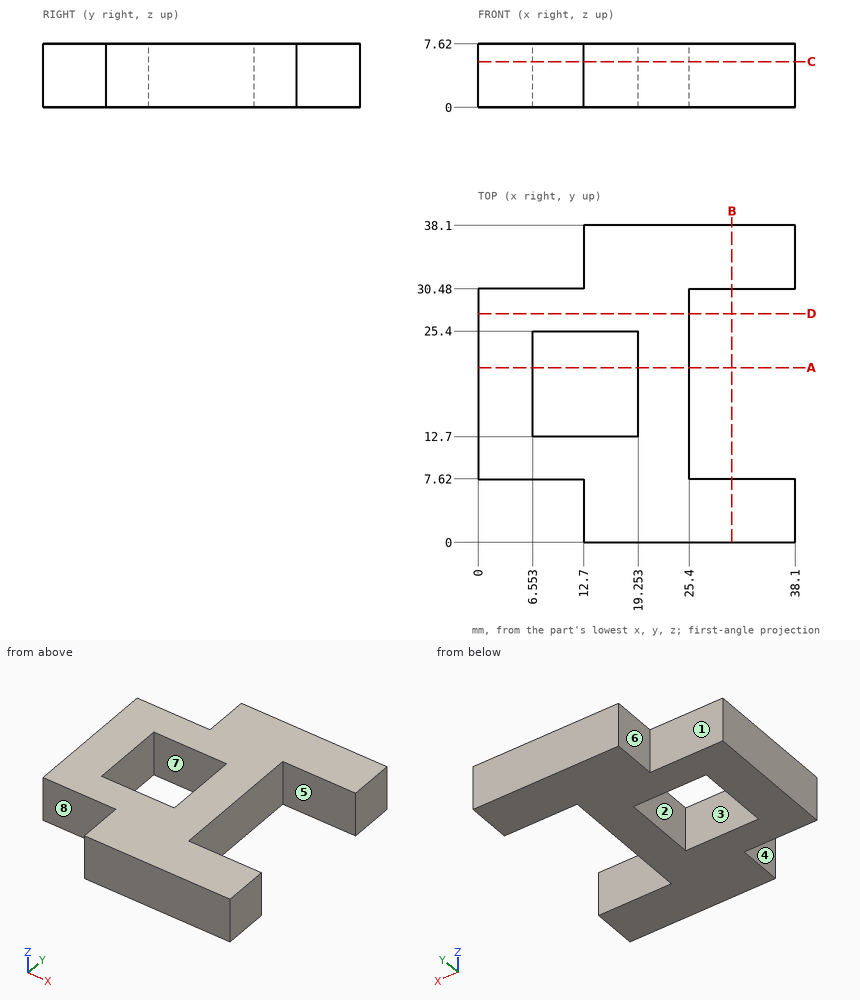
Input: dimensioned drawing with shaded views. Units: mm. Origin: part minimum x, y, z. A direction names the side the tool comes from. Give positions to 0.01 mm unless a question says otherwise; leave off trailing zeros. Loops run counter-clockwise (first coordinate to the right, second up) from the corner with the lowest first, then second, coordinate; pieces in that order, holes last. Notation, with made-up numbers: M 18,-10 L 63,-10 A33 ccw 63,23 Z; hole C 82,42.5 d11. An arc over 180 degrees is marked long. Put each result on its own line as item: value. Start each with the question number.
1) Ray query, line 1 along Y through (x, z) = (9, 6); line 2 along X through (y, z) = (13.5, 5); line 3 along Y through (x, z) = (36, 4). Return the intervals inside material, ascending.
2) Contact query for flat-ended pins moving along their axis: pin 1 (10 mm diameter, centred on x = 24, y = 8.5, fed in from -Z); pin 2 (2.5 mm diameter, centred on x = 6, z = 4.5, fed in from -Y); pin 3 (2.5 mm diameter, centred on y = 21.5, z = 2.5, fed in from +X); pin 4 (4 mm diameter, centred on y = 5.5, z = 5.5, fed in from -X). Output: stop coordinate, or through.
3) Access query for the marked faces 5, 6, 7 and 8. Directions: +Z, -Z, +X, -X, +Y, -Y. A direction counts if a zero-diameter tool reaches every point of the face in a straight line with its end or side. Return the directions, or none.
4) Pull-direction query (X, two-part tool) for the marked faces 1, 2, 3 and 4; classes: pulls with the +X half, pulls with the -X half, needs draft (parallel to the pull), parting line crosses it, or undercut.
5) Cut plane B-B (x = 30.5). Output: boundary loops of the cut face in (y, z), then the cut area to 3 significant figures.
6) Cut plane D-D (y = 27.5). Output: boundary loops of the cut face in (x, z).
7) Cut plane A-A (y = 21). Output: boundary loops of the cut face in (x, z), then the cut area to 3 significant figures.
8) Cut plane C-C (z = 5.5). Output: boundary loops of the cut face in (x, y).
Verdict:
1. line 1: 7.62 to 12.7, 25.4 to 30.48
1. line 2: 0 to 6.55, 19.25 to 25.4
1. line 3: 0 to 7.62, 30.48 to 38.1
2. pin 1: z = 0
2. pin 2: y = 7.62
2. pin 3: x = 25.4
2. pin 4: x = 12.7
3. face 5: +Z, -Z, +X
3. face 6: +Z, -Z, -X, +Y
3. face 7: +Z, -Z
3. face 8: +Z, -Z, -X, -Y
4. face 1: needs draft
4. face 2: undercut
4. face 3: undercut
4. face 4: pulls with the -X half
5. outline: M 0,0 L 7.62,0 L 7.62,7.62 L 0,7.62 Z; M 30.48,0 L 38.1,0 L 38.1,7.62 L 30.48,7.62 Z
5. area: 116 mm2
6. outline: M 0,0 L 25.4,0 L 25.4,7.62 L 0,7.62 Z
7. outline: M 0,0 L 6.55,0 L 6.55,7.62 L 0,7.62 Z; M 19.25,0 L 25.4,0 L 25.4,7.62 L 19.25,7.62 Z
7. area: 96.8 mm2
8. outline: M 0,7.62 L 12.7,7.62 L 12.7,0 L 38.1,0 L 38.1,7.62 L 25.4,7.62 L 25.4,30.48 L 38.1,30.48 L 38.1,38.1 L 12.7,38.1 L 12.7,30.48 L 0,30.48 Z; hole M 6.55,12.7 L 19.25,12.7 L 19.25,25.4 L 6.55,25.4 Z
